from build123d import *

# Parameters (mm, degrees)
SKETCH008_R                               = 9.069179
SKETCH008_R_2                             = 1
EXTRUDE009_DEPTH                          = 1
SKETCH007_R                               = 9.069179
SKETCH007_R_2                             = 1
EXTRUDE008_DEPTH                          = 1
SKETCH006_AS_DRAWN_R                      = 9.069179
SKETCH006_AS_DRAWN_R_2                    = 1
EXTRUDE007_DEPTH                          = 1
EXTRUDE007_ONTO_SKETCH006_ROLL_ANGLE      = 90
EXTRUDE007_ONTO_SKETCH006_PLACEMENT_ANGLE = 180
SKETCH005_R                               = 9.069179
SKETCH005_R_2                             = 1
EXTRUDE006_DEPTH                          = 1
SKETCH004_AS_DRAWN_R                      = 9.069179
SKETCH004_AS_DRAWN_R_2                    = 1
EXTRUDE005_DEPTH                          = 1
EXTRUDE005_ONTO_SKETCH004_ROLL_ANGLE      = 90
SKETCH003_R                               = 1
EXTRUDE004_DEPTH                          = 1
SKETCH002_R                               = 9.069179
EXTRUDE_DEPTH                             = 1
SKETCH001_W                               = 20
SKETCH001_H                               = 20
EXTRUDE003_DEPTH                          = 20
CHAMFER_SIZE2                             = 0.57
CHAMFER_SIZE                              = 0.99
CHAMFER001_SIZE2                          = 0.57
CHAMFER001_SIZE                           = 0.99
CHAMFER002_SIZE2                          = 0.57
CHAMFER002_SIZE                           = 0.99
CHAMFER003_SIZE2                          = 0.99
CHAMFER003_SIZE                           = 0.57
CHAMFER004_SIZE2                          = 0.57
CHAMFER004_SIZE                           = 0.99
CHAMFER005_SIZE2                          = 0.99
CHAMFER005_SIZE                           = 0.57
CHAMFER006_SIZE2                          = 0.57
CHAMFER006_SIZE                           = 0.99
CHAMFER007_SIZE2                          = 0.99
CHAMFER007_SIZE                           = 0.57
CHAMFER008_SIZE2                          = 0.57
CHAMFER008_SIZE                           = 0.99
CHAMFER009_SIZE2                          = 0.99
CHAMFER009_SIZE                           = 0.57
CHAMFER010_SIZE2                          = 0.57
CHAMFER010_SIZE                           = 0.99
CHAMFER011_SIZE2                          = 0.99
CHAMFER011_SIZE                           = 0.57


with BuildPart() as extrude009:
    # Sketch008 → Extrude009 (new body)
    with BuildSketch(Plane(origin=(0, 0, 0), x_dir=(1, 0, 0), z_dir=(0, 0, -1))):
        Circle(SKETCH008_R)
        with Locations((-3.5, 5)):
            Circle(SKETCH008_R_2, mode=Mode.SUBTRACT)
        with Locations((-3.5, -5)):
            Circle(SKETCH008_R_2, mode=Mode.SUBTRACT)
        with Locations((3.5, -5)):
            Circle(SKETCH008_R_2, mode=Mode.SUBTRACT)
        with Locations((3.5, 5)):
            Circle(SKETCH008_R_2, mode=Mode.SUBTRACT)
        with Locations((-3.5, 0)):
            Circle(SKETCH008_R_2, mode=Mode.SUBTRACT)
        with Locations((3.5, 0)):
            Circle(SKETCH008_R_2, mode=Mode.SUBTRACT)
    extrude(amount=-EXTRUDE009_DEPTH)


with BuildPart() as extrude008:
    # Sketch007 → Extrude008 (new body)
    with BuildSketch(Plane(origin=(-10, 0, 0), x_dir=(0, -1, 0), z_dir=(-1, 0, 0))):
        with Locations((0, 10)):
            Circle(SKETCH007_R)
        with Locations((3.535534, 13.535534)):
            Circle(SKETCH007_R_2, mode=Mode.SUBTRACT)
        with Locations((-3.535534, 6.464466)):
            Circle(SKETCH007_R_2, mode=Mode.SUBTRACT)
    extrude(amount=-EXTRUDE008_DEPTH)


with BuildPart() as extrude007:
    # Sketch006 as drawn → Extrude007 (new)
    with BuildSketch(Plane.XY):
        with Locations((0, 10)):
            Circle(SKETCH006_AS_DRAWN_R)
        with Locations((-3.535534, 13.535534)):
            Circle(SKETCH006_AS_DRAWN_R_2, mode=Mode.SUBTRACT)
        with Locations((3.535534, 13.535534)):
            Circle(SKETCH006_AS_DRAWN_R_2, mode=Mode.SUBTRACT)
        with Locations((3.535534, 6.464466)):
            Circle(SKETCH006_AS_DRAWN_R_2, mode=Mode.SUBTRACT)
        with Locations((-3.535534, 6.464466)):
            Circle(SKETCH006_AS_DRAWN_R_2, mode=Mode.SUBTRACT)
    extrude(amount=-EXTRUDE007_DEPTH)


with BuildPart() as extrude007_1:
    # Extrude007 onto Sketch006 roll: moved
    add(extrude007.part.rotate(Axis((0, 0, 0), (1, 0, 0)), EXTRUDE007_ONTO_SKETCH006_ROLL_ANGLE))


with BuildPart() as extrude007_2:
    # Extrude007 onto Sketch006 placement: moved
    add(extrude007_1.part.moved(Location((0, 10, 0))).rotate(Axis((0, 10, 0), (0, 0, 1)), EXTRUDE007_ONTO_SKETCH006_PLACEMENT_ANGLE))


with BuildPart() as extrude006:
    # Sketch005 → Extrude006 (new body)
    with BuildSketch(Plane.YZ.offset(10)):
        with Locations((0, 10)):
            Circle(SKETCH005_R)
        with Locations((0, 10)):
            Circle(SKETCH005_R_2, mode=Mode.SUBTRACT)
        with Locations((-3.535534, 6.464466)):
            Circle(SKETCH005_R_2, mode=Mode.SUBTRACT)
        with Locations((-3.535534, 13.535534)):
            Circle(SKETCH005_R_2, mode=Mode.SUBTRACT)
        with Locations((3.535534, 13.535534)):
            Circle(SKETCH005_R_2, mode=Mode.SUBTRACT)
        with Locations((3.535534, 6.464466)):
            Circle(SKETCH005_R_2, mode=Mode.SUBTRACT)
    extrude(amount=-EXTRUDE006_DEPTH)


with BuildPart() as extrude005:
    # Sketch004 as drawn → Extrude005 (new)
    with BuildSketch(Plane.XY):
        with Locations((0, 10)):
            Circle(SKETCH004_AS_DRAWN_R)
        with Locations((0, 10)):
            Circle(SKETCH004_AS_DRAWN_R_2, mode=Mode.SUBTRACT)
        with Locations((3.535534, 13.535534)):
            Circle(SKETCH004_AS_DRAWN_R_2, mode=Mode.SUBTRACT)
        with Locations((-3.535534, 6.464466)):
            Circle(SKETCH004_AS_DRAWN_R_2, mode=Mode.SUBTRACT)
    extrude(amount=-EXTRUDE005_DEPTH)


with BuildPart() as extrude005_1:
    # Extrude005 onto Sketch004 roll: moved
    add(extrude005.part.rotate(Axis((0, 0, 0), (1, 0, 0)), EXTRUDE005_ONTO_SKETCH004_ROLL_ANGLE))


with BuildPart() as extrude005_2:
    # Extrude005 onto Sketch004 placement: moved
    add(extrude005_1.part.moved(Location((0, -10, 0))))


with BuildPart() as extrude004:
    # Sketch003 → Extrude004 (new body)
    with BuildSketch(Plane.XY.offset(19)):
        Circle(SKETCH003_R)
    extrude(amount=EXTRUDE004_DEPTH)


with BuildPart() as extrude_body:
    # Sketch002 → Extrude (new body)
    with BuildSketch(Plane.XY.offset(20)):
        Circle(SKETCH002_R)
    extrude(amount=-EXTRUDE_DEPTH)


with BuildPart() as extrude003:
    # Sketch001 → Extrude003 (new body)
    with BuildSketch(Plane.XY):
        Rectangle(SKETCH001_W, SKETCH001_H)
    extrude(amount=EXTRUDE003_DEPTH)


with BuildPart() as chamfer011:
    # Sketch → Revolve (revolve)
    with BuildSketch(Plane.XY):
        with BuildLine():
            ThreePointArc((0, -13.5), (13.5, 0), (0, 13.5))
            Line((0, 13.5), (0, -13.5))
        make_face()
    revolve(axis=Axis((0, 0, 0), (0, 1, 0)))


with BuildPart() as chamfer011_1:
    # Revolve placement: moved
    add(chamfer011.part.moved(Location((0, 0, 10))))

    # Common: intersect Extrude003
    add(extrude003.part, mode=Mode.INTERSECT)

    # Cut: cut Extrude body
    add(extrude_body.part, mode=Mode.SUBTRACT)

    # Chamfer
    chamfer_edges = [chamfer011_1.edges().sort_by_distance(p)[0] for p in [
        (-9.069179, 0, 19),
    ]]
    chamfer_side = chamfer011_1.faces().sort_by_distance((-9.069179, 0, 19.5))[0]
    chamfer(chamfer_edges, length=CHAMFER_SIZE, length2=CHAMFER_SIZE2, reference=chamfer_side)

    # Fusion: union Extrude004
    add(extrude004.part)

    # Chamfer001
    chamfer001_edges = [chamfer011_1.edges().sort_by_distance(p)[0] for p in [
        (-1, 0, 19),
    ]]
    chamfer001_side = chamfer011_1.faces().sort_by_distance((-1, 0, 19.5))[0]
    chamfer(chamfer001_edges, length=CHAMFER001_SIZE, length2=CHAMFER001_SIZE2, reference=chamfer001_side)

    # Cut001: cut Extrude005
    add(extrude005_2.part, mode=Mode.SUBTRACT)

    # Chamfer002
    chamfer002_edges = [chamfer011_1.edges().sort_by_distance(p)[0] for p in [
        (-9.069179, -9, 10),
    ]]
    chamfer002_side = chamfer011_1.faces().sort_by_distance((-9.069179, -9.5, 10))[0]
    chamfer(chamfer002_edges, length=CHAMFER002_SIZE, length2=CHAMFER002_SIZE2, reference=chamfer002_side)

    # Chamfer003
    chamfer003_edges = [chamfer011_1.edges().sort_by_distance(p)[0] for p in [
        (2.535534, -9, 13.535534),
        (-1, -9, 10),
        (-4.535534, -9, 6.464466),
    ]]
    chamfer003_side = chamfer011_1.faces().sort_by_distance((-8.258786, -9, 10))[0]
    chamfer(chamfer003_edges, length=CHAMFER003_SIZE, length2=CHAMFER003_SIZE2, reference=chamfer003_side)

    # Cut002: cut Extrude006
    add(extrude006.part, mode=Mode.SUBTRACT)

    # Chamfer004
    chamfer004_edges = [chamfer011_1.edges().sort_by_distance(p)[0] for p in [
        (9, -9.069179, 10),
    ]]
    chamfer004_side = chamfer011_1.faces().sort_by_distance((9.5, -9.069179, 10))[0]
    chamfer(chamfer004_edges, length=CHAMFER004_SIZE, length2=CHAMFER004_SIZE2, reference=chamfer004_side)

    # Chamfer005
    chamfer005_edges = [chamfer011_1.edges().sort_by_distance(p)[0] for p in [
        (9, 2.535534, 13.535534),
        (9, -4.535534, 13.535534),
        (9, -1, 10),
        (9, 2.535534, 6.464466),
        (9, -4.535534, 6.464466),
    ]]
    chamfer005_side = chamfer011_1.faces().sort_by_distance((9, -8.258786, 10))[0]
    chamfer(chamfer005_edges, length=CHAMFER005_SIZE, length2=CHAMFER005_SIZE2, reference=chamfer005_side)

    # Cut003: cut Extrude007
    add(extrude007_2.part, mode=Mode.SUBTRACT)

    # Chamfer006
    chamfer006_edges = [chamfer011_1.edges().sort_by_distance(p)[0] for p in [
        (9.069179, 9, 10),
    ]]
    chamfer006_side = chamfer011_1.faces().sort_by_distance((9.069179, 9.5, 10))[0]
    chamfer(chamfer006_edges, length=CHAMFER006_SIZE, length2=CHAMFER006_SIZE2, reference=chamfer006_side)

    # Chamfer007
    chamfer007_edges = [chamfer011_1.edges().sort_by_distance(p)[0] for p in [
        (-2.535534, 9, 13.535534),
        (4.535534, 9, 13.535534),
        (4.535534, 9, 6.464466),
        (-2.535534, 9, 6.464466),
    ]]
    chamfer007_side = chamfer011_1.faces().sort_by_distance((0, 9, 10))[0]
    chamfer(chamfer007_edges, length=CHAMFER007_SIZE, length2=CHAMFER007_SIZE2, reference=chamfer007_side)

    # Cut004: cut Extrude008
    add(extrude008.part, mode=Mode.SUBTRACT)

    # Chamfer008
    chamfer008_edges = [chamfer011_1.edges().sort_by_distance(p)[0] for p in [
        (-9, 9.069179, 10),
    ]]
    chamfer008_side = chamfer011_1.faces().sort_by_distance((-9.5, 9.069179, 10))[0]
    chamfer(chamfer008_edges, length=CHAMFER008_SIZE, length2=CHAMFER008_SIZE2, reference=chamfer008_side)

    # Chamfer009
    chamfer009_edges = [chamfer011_1.edges().sort_by_distance(p)[0] for p in [
        (-9, -2.535534, 13.535534),
        (-9, 4.535534, 6.464466),
    ]]
    chamfer009_side = chamfer011_1.faces().sort_by_distance((-9, 0, 10))[0]
    chamfer(chamfer009_edges, length=CHAMFER009_SIZE, length2=CHAMFER009_SIZE2, reference=chamfer009_side)

    # Cut005: cut Extrude009
    add(extrude009.part, mode=Mode.SUBTRACT)

    # Chamfer010
    chamfer010_edges = [chamfer011_1.edges().sort_by_distance(p)[0] for p in [
        (-9.069179, 0, 1),
    ]]
    chamfer010_side = chamfer011_1.faces().sort_by_distance((-9.069179, 0, 0.5))[0]
    chamfer(chamfer010_edges, length=CHAMFER010_SIZE, length2=CHAMFER010_SIZE2, reference=chamfer010_side)

    # Chamfer011
    chamfer011_edges = [chamfer011_1.edges().sort_by_distance(p)[0] for p in [
        (2.5, -5, 1),
        (2.5, 0, 1),
        (-4.5, 0, 1),
        (2.5, 5, 1),
        (-4.5, 5, 1),
        (-4.5, -5, 1),
    ]]
    chamfer011_side = chamfer011_1.faces().sort_by_distance((0, 0, 1))[0]
    chamfer(chamfer011_edges, length=CHAMFER011_SIZE, length2=CHAMFER011_SIZE2, reference=chamfer011_side)


solid = chamfer011_1.part
Design review of the part built by this model. Coordinates are the model's own, in mm. Round coordinates to 2 decimals unless told otherwise and drop trailing zeros. Answer as CSV lines item,"result". Start each with the question number.
1) The part is to be moulded in two halves that separate along X. For faces 1 (the face through (2, -9, 10)), 2 (the face through (-4, 10, 6)), 3 (the face through (10, 0, 10)), say which applies: +X half, -X half, draft (parallel to the pull), parting line (faces both ways), or undercut.
2) Wall thickness on line 1 along Y through (x, z) = (-7, 13.5); line 2 along Z through (x, y) = (6.5, -4.75): over which ranges is each line inside the solid? List them lowest first. Write a range as [from, to].
3) For pin 1 Ø2 at (y, z) = (-5, 7.5) entering from -X; pin 2 Ø2 at (y, z) = (3.5, 9.5) entering from +X, all flat-tipped, find the tip position at first contact; note any pin that passes through.
Resolved:
1,face 1,"undercut"
1,face 2,"draft"
1,face 3,"+X half"
2,line 1,"[-9, 9]"
2,line 2,"[1, 19]"
3,pin 1,"x = -9"
3,pin 2,"x = 9"
